Build history of the part. All positions in model axes, mm. A direction names the side the tool comes from. Round coordinates to 2 decimals unless told otherwise and drop trailing zeros. Write each loop counter-clockwise with the first axis right and the second up, starting at its lowest first coordinate (ties: lowest second). Pieces come first, ordered by that corner, then holes.
Item 1: Mould opens along Z. For faces 3 (the flat face through (2, 0, -13)), 4 (the cylindrical face through (1.61, 20.42, -50.54)), 5 (the cylindrical face through (1.57, 1.81, -1.91)), 6 (the cylindrical face through (1.61, 46.842, -12.386)) say: +Z half, -Z half, draft (parallel to the pull), parting line (faces both ways), or undercut.
Item 2: Band-saw the part on B-B, the plane y = 17. Write the cut outline in (x, z) (3 decimals), then the cut area to 3 significant figures.
Item 3: Band-saw the part on C-C, the plane x = 1.15. Write the cut outline in (y, z), then the cut area to 3 significant figures.
Item 4: Band-saw the part on A-A, the plane z = -12.7. Write the cut outline in (x, y) (3 decimals).
Item 5: Wall check: probe 1 along Y at (x, z) = (0.9, -12.5); probe 2 along Z at (x, y) = (2.4, 45.5); probe 3 along Z at (x, y) = (1.4, 11.5). Give the ranges that are in metal, low to high.
Item 6: 3-axis set-ups, long thin cutter, end or side, ignore diameter. For faces 1 (the flat face through (1.565, 11.823, -54.199)), 2 (the flat face through (1.57, 12.88, -38.59)): which of +Z, -Z, +X, -X, +Y, -Y reach the whole face in a straight line?
Item 7: Drop a flat-ended pin along its axis: pin 1 Ø1.5 at (y, z) = (33, -14.5) entering from -X. Give the stop position or say it passes through.
Item 8: Band-saw the part on D-D, the plane y = 44.45. Write the cut outline in (x, z) (3 decimals), then the cut area to 3 significant figures.
```python
from build123d import *

# Parameters (mm, degrees)
BOSS_EXTRUDE1_DEPTH = 3.175
SKETCH2_R           = 2.413
CUT_EXTRUDE1_DEPTH  = 105.401092279


with BuildPart() as part:
    # Sketch1 → Boss-Extrude1 (new body)
    with BuildSketch(Plane(origin=(0, 0, 0), x_dir=(0, 0, -1), z_dir=(1, 0, 0))):
        with BuildLine():
            Line((27.254915981, 80.437799327), (61.677992598, 23.799518102))
            ThreePointArc((61.677992598, 23.799518102), (62.420677668, 18.996519818), (59.549602661, 15.075129511))
            Line((59.549602661, 15.075129511), (48.696824135, 8.479130857))
            ThreePointArc((48.696824135, 8.479130857), (43.89382585, 7.736445787), (39.972435544, 10.607520794))
            Line((39.972435544, 10.607520794), (37.176389263, 15.208017644))
            ThreePointArc((37.176389263, 15.208017644), (30.037556106, 18.024757552), (25.4, 11.910018317))
            Line((25.4, 11.910018317), (25.4, 6.35))
            ThreePointArc((25.4, 6.35), (23.540128061, 1.859871939), (19.05, 0))
            Line((19.05, 0), (6.35, 0))
            ThreePointArc((6.35, 0), (1.859871939, 1.859871939), (0, 6.35))
            Line((0, 6.35), (0, 77.1398))
            ThreePointArc((0, 77.1398), (1.859871939, 81.629928061), (6.35, 83.4898))
            Line((6.35, 83.4898), (21.828526718, 83.4898))
            ThreePointArc((21.828526718, 83.4898), (24.941419607, 82.674454268), (27.254915981, 80.437799327))
        make_face()
    extrude(amount=BOSS_EXTRUDE1_DEPTH)

    # Sketch2 → Cut-Extrude1 (cut, through all)
    with BuildSketch(Plane(origin=(3.175, 0, 0), x_dir=(0, 0, -1), z_dir=(1, 0, 0))):
        with Locations((12.7, 12.7)):
            Circle(SKETCH2_R)
        with Locations((12.7, 44.45)):
            Circle(SKETCH2_R)
        with Locations((12.7, 69.85)):
            Circle(SKETCH2_R)
        with Locations((34.821609996, 43.535175921)):
            Circle(SKETCH2_R)
        with Locations((48.30950313, 21.342764331)):
            Circle(SKETCH2_R)
    extrude(amount=-CUT_EXTRUDE1_DEPTH, mode=Mode.SUBTRACT)


solid = part.part
```
Results:
1. face 3: draft
1. face 4: undercut
1. face 5: +Z half
1. face 6: undercut
2. outline: (0, -61.549) - (3.175, -61.549) - (3.175, -35.547) - (0, -35.547) - close; (0, -27.953) - (3.175, -27.953) - (3.175, 0) - (0, 0) - close
2. area: 171 mm2
3. outline: (0, -19.05) arc R6.35 ccw to (6.35, -25.4) - (11.91, -25.4) arc R6.35 cw to (15.21, -37.18) - (10.61, -39.97) arc R6.35 ccw to (8.48, -48.7) - (15.08, -59.55) arc R6.35 ccw to (23.8, -61.68) - (80.44, -27.25) arc R6.35 ccw to (83.49, -21.83) - (83.49, -6.35) arc R6.35 ccw to (77.14, 0) - (6.35, 0) arc R6.35 ccw to (0, -6.35) - close; hole circle Ø4.83 at (12.7, -12.7); hole circle Ø4.83 at (21.34, -48.31); hole circle Ø4.83 at (43.54, -34.82); hole circle Ø4.83 at (44.45, -12.7); hole circle Ø4.83 at (69.85, -12.7)
3. area: 3,480 mm2
4. outline: (0, 0) - (3.175, 0) - (3.175, 10.287) - (0, 10.287) - close; (0, 15.113) - (3.175, 15.113) - (3.175, 42.037) - (0, 42.037) - close; (0, 46.863) - (3.175, 46.863) - (3.175, 67.437) - (0, 67.437) - close; (0, 72.263) - (3.175, 72.263) - (3.175, 83.49) - (0, 83.49) - close
5. probe 1: y = 0 to 10.3, 15.1 to 42.05, 46.85 to 67.45, 72.25 to 83.49
5. probe 2: z = -48.49 to -36.22, -33.42 to -14.87, -10.53 to 0
5. probe 3: z = -53.67 to -39.43, -25.4 to -14.79, -10.61 to 0
6. face 1: -Z, +X, -X, -Y
6. face 2: +X, -X, -Y
7. pin 1: stops at x = 0
8. outline: (0, -49.127) - (3.175, -49.127) - (3.175, -37.054) - (0, -37.054) - close; (0, -32.589) - (3.175, -32.589) - (3.175, -15.113) - (0, -15.113) - close; (0, -10.287) - (3.175, -10.287) - (3.175, 0) - (0, 0) - close
8. area: 126 mm2
